Autodesk Inventor part; units mm, degrees
ref_plane "YZ Plane" through (0, 0, 0) normal (1, 0, 0) x (0, 1, 0)
ref_plane "XZ Plane" through (0, 0, 0) normal (0, 1, 0) x (-1, 0, 0)
ref_plane "XY Plane" through (0, 0, 0) normal (0, 0, 1) x (1, 0, 0)
sketch "Sketch1" plane through (0, 0, 0) normal (0, 0, 1) x (1, 0, 0)
  line L0 (-68.6002, -120.3249) -> (31.3998, -120.3249)
  line L1 (31.3998, -120.3249) -> (31.3998, 129.6751)
  line L2 (31.3998, 129.6751) -> (11.3998, 129.6751)
  line L3 (11.3998, 129.6751) -> (11.3998, 84.6751)
  line L4 (11.3998, 84.6751) -> (-58.6002, 81.0066)
  line L5 (-68.6002, -120.3249) -> (-68.6002, 77.725)
  line L6 (-68.6002, 77.725) -> (-68.6002, 129.6751)
  line L7 (-68.6002, 129.6751) -> (-58.6002, 129.6751)
  line L8 (-58.6002, 129.6751) -> (-58.6002, 81.0066)
  line L9 (31.3998, -120.3249) -> (41.3973, -120.3249) construction
  line L10 (31.3998, 4.6751) -> (-68.6002, 4.6751) construction
  line L11 (31.3998, 4.6751) -> (36.4024, 4.6751)
  line L12 (36.4024, 14.8241) -> (31.3973, 14.8241)
  line L13 (31.3973, 14.8241) -> (31.3998, 4.6751)
  line L14 (-68.6002, 129.6751) -> (-68.6002, 79.6751)
  line L15 (-68.6002, 79.6751) -> (31.3998, 79.6751) construction
  line L16 (36.3973, 114.8241) -> (31.3973, 114.8241)
  line L17 (31.3973, 104.7241) -> (36.3973, 104.7241)
  line L18 (36.3973, -85.1759) -> (31.3973, -85.1759)
  line L19 (31.3973, -95.2759) -> (36.3973, -95.2759)
  line L20 (36.4024, 14.8241) -> (31.4024, 14.8241)
  line L21 (31.4024, 4.7241) -> (36.4024, 4.7241)
  line L22 (-18.6002, -120.3249) -> (-18.6002, 129.7241) construction
  line L23 (-73.6027, 14.8241) -> (-68.5976, 14.8241)
  line L24 (-73.6027, 14.8241) -> (-68.6027, 14.8241)
  line L25 (-68.6002, 4.6751) -> (-73.6027, 4.6751)
  line L26 (-68.6027, 4.7241) -> (-73.6027, 4.7241)
  line L27 (-73.6027, 4.6751) -> (-73.6027, 14.8241)
  line L28 (-73.6027, 4.7241) -> (-73.6027, 14.8241)
  line L29 (-73.5976, -85.1759) -> (-68.5976, -85.1759)
  line L30 (-73.5976, -95.2759) -> (-73.5976, -85.1759)
  line L31 (-68.5976, -95.2759) -> (-73.5976, -95.2759)
  line L32 (-68.6002, -120.3249) -> (-78.6002, -120.3249)
  line L33 (-58.6002, 81.0066) -> (-68.6002, 81.0556) construction
  line L34 (36.4024, 14.8241) -> (36.4024, 4.7241)
  line L35 (36.3973, 114.8241) -> (36.3973, 104.7241)
  line L36 (36.3973, -85.1759) -> (36.3973, -95.2759)
  line L37 (11.2345, 78.6582) -> (0.2496, 78.0825)
  line L38 (0.2496, 78.0825) -> (-0.0644, 84.0743)
  line L39 (-0.0644, 84.0743) -> (10.9205, 84.65)
  line L40 (10.9205, 84.65) -> (11.2345, 78.6582)
  line L41 (-57.9849, 81.0388) -> (10.9205, 84.65)
  line L42 (-57.6709, 75.047) -> (-57.9849, 81.0388)
  line L43 (-46.686, 75.6227) -> (-57.6709, 75.047)
  line L44 (-47, 81.6145) -> (-46.686, 75.6227)
  point P0 (0, 0)
  point P1 (21.3998, 129.6751)
  point P2 (-63.6002, 129.6751)
  point P3 (-68.6002, 14.8241)
  point P4 (-68.6002, 4.6751)
  point P5 (-68.6002, -85.1759)
  point P6 (-68.6002, -95.2759)
  point P7 (31.3998, -95.2759)
  point P8 (31.3998, -85.1759)
  point P9 (36.3973, 4.7241)
  point P10 (36.4024, 14.8241)
  point P11 (31.3998, 14.8241)
  point P12 (31.3998, 104.7241)
  point P13 (31.3998, 114.8241)
  dimension "d0" = 100
  dimension "d2" = 20
  dimension "d4" = 93
  dimension "d5" = 10
  dimension "d6" = 85
  dimension "d10" = 50
  dimension "d12" = 100
  dimension "d13" = 10
  dimension "d33" = 11
  dimension "d34" = 6
  dimension "d35" = 10
  dimension "d36" = 11
  dimension "d37" = 6
  dimension "d43" = 0
extrude "Extrusion1" add sketch "Sketch1" along normal blind 5
properties part number "Lifting Sections leftt"
Geometry: final body of the model. Coordinates: model frame, mm. A direction names the side the tool comes from. Coordinates: 2 decimals unless noted, no trailing zeros. Write each loop counter-clockwise with the first axis right and the second up, starting at its lowest first coordinate (ties: lowest second). Pieces come first, ordered by that corner, then holes. Notation, with made-up numbers: M 12.25,86.5 L 21.25,86.5 A29 cw 21.25,121.5 Z; hole C 7,72 d4. An arc over 180 degrees is marked long. Use CSV: the item, a comma, the result in double quotes. Start each with the question number.
1. Cut plane D-D on x = -41. Return the cut outline in (y, z).
2. Mould query, pull axis Y, two halves, no side actions, for faces 6 (the face through (22, 129.675, 2)), 7 (the face through (-73.598, -90, 2)), 8 (the face through (-71, -85.176, 2)). Classes: pulls with the +Y half, pulls with the -Y half, needs draft (parallel to the pull), parting line crosses it, or undercut.
3. First-contact query: P1, Ø2.5, axis at y = 121.5, z = 2.5, coming from the +X side; P2, Ø1.5, axis at x = 34.5, z = 3.5, coming from the -Y side; P3, Ø2.5, axis at x = 33, z = 2.5, coming from the +Y side. Flat tips, straight axial feed; report the tip coordinate or a pass-through.
4. Cut plane C-C on y = -63. Return the cut outline in (x, z).
5. Ray query, probe 1 along X at (y, z) = (99.5, 0.4); probe 2 along X at (y, z) = (39.5, 1.85); probe 3 along Y at (x, z) = (-7, 3.5). Return the intervals inside material, ascending.
6. Cut plane B-B on z = 4.1. Return the cut outline in (x, y).
7. Reachability of faces 1 (the face through (31.4, 8, 2)), 2 (the face through (34, -95.276, 2)), 3 (the face through (-71, 14.824, 2)), 4 (the face through (-68.6, -108, 2)), 5 (the face through (11.4, 107, 2)) from +Z, -Z, +X, -X, +Y, -Y: full face, straight path, thin tool, end or side. Return the list, or none.
8. Cut plane A-A on y = 95.5. Return the cut outline in (x, z).
Entries:
1,outline,"M -120.32,0 L 81.93,0 L 81.93,5 L -120.32,5 Z"
2,face 6,"pulls with the +Y half"
2,face 7,"needs draft"
2,face 8,"undercut"
3,P1,"x = 31.4"
3,P2,"y = -95.28"
3,P3,"y = 114.82"
4,outline,"M -68.6,0 L 31.4,0 L 31.4,5 L -68.6,5 Z"
5,probe 1,"-68.6 to -58.6, 11.4 to 31.4"
5,probe 2,"-68.6 to 31.4"
5,probe 3,"-120.32 to 83.71"
6,outline,"M -73.6,-95.28 L -68.6,-95.28 L -68.6,-120.32 L 31.4,-120.32 L 31.4,-95.28 L 36.4,-95.28 L 36.4,-85.18 L 31.4,-85.18 L 31.4,104.72 L 36.4,104.72 L 36.4,114.82 L 31.4,114.82 L 31.4,129.68 L 11.4,129.68 L 11.4,84.68 L -58.6,81.01 L -58.6,129.68 L -68.6,129.68 L -68.6,14.82 L -73.6,14.82 L -73.6,4.68 L -68.6,4.68 L -68.6,-85.18 L -73.6,-85.18 Z"
7,face 1,"+Z, -Z, +X"
7,face 2,"+Z, -Z, +X, -Y"
7,face 3,"+Z, -Z, -X, +Y"
7,face 4,"+Z, -Z, -X, -Y"
7,face 5,"+Z, -Z, +Y"
8,outline,"M -68.6,0 L -58.6,0 L -58.6,5 L -68.6,5 Z; M 11.4,0 L 31.4,0 L 31.4,5 L 11.4,5 Z"
